Geometry: final body of the model. Coordinates: model frame, mm. Face numbers are marked on the shaded views. A direction names the side the tool comes from. Round coordinates to 2 decimals unless told otherwise and drop trailing zeros. Loops run counter-clockwise (first coordinate to the right, second up) from the corner with the lowest first, then second, coordinate; pieces in that order, holes last. Notation, with made-up numbers: M -4.5,71.5 L 33.5,71.5 A12 ccw 33.5,87.5 Z; hole C 5.25,53 d3. An arc over 180 degrees is marked long. Answer as a JSON object with one key per item and string values.
from build123d import *

# Parameters (mm, degrees)
F1_DEPTH = 6.35


with BuildPart() as f1:
    # F0 (on Front) → F1 (new body)
    with BuildSketch(Plane.XZ):
        with BuildLine():
            Line((52.175445, 0), (0, 0))
            ThreePointArc((0, 0), (-4.7752, -4.7752), (0, -9.5504))
            Line((0, -9.5504), (52.175445, -9.5504))
            ThreePointArc((52.175445, -9.5504), (54.631508, -10.044612), (56.705267, -11.45032))
            ThreePointArc((56.705267, -11.45032), (63.5, -14.3002), (70.294733, -11.45032))
            ThreePointArc((70.294733, -11.45032), (70.729047, -10.49401), (70.294733, -9.5377))
            Line((70.294733, -9.5377), (63.5, -9.5377))
            ThreePointArc((63.5, -9.5377), (58.7375, -4.7752), (63.5, -0.0127))
            Line((63.5, -0.0127), (70.294733, -0.0127))
            ThreePointArc((70.294733, -0.0127), (70.729047, 0.94361), (70.294733, 1.89992))
            ThreePointArc((70.294733, 1.89992), (63.5, 4.7498), (56.705267, 1.89992))
            ThreePointArc((56.705267, 1.89992), (54.631508, 0.494212), (52.175445, 0))
        make_face()
    extrude(amount=F1_DEPTH)


solid = f1.part
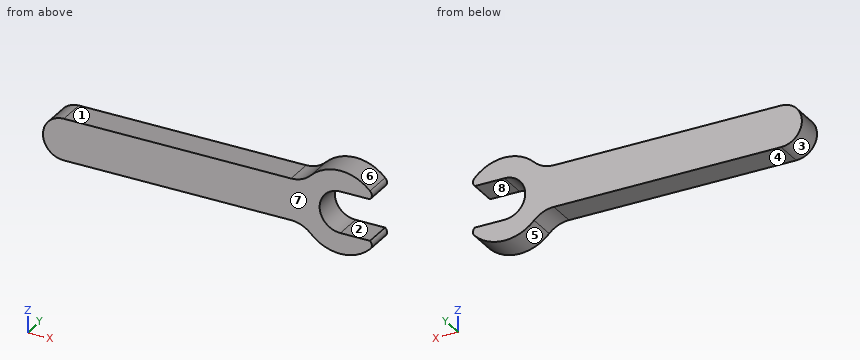
1) Ray query, line 1 (Z direction, x = 64, y = -1.75); line 2 (Z direction, x = 5, y = -0.75); line 3 (Z direction, x = 61, y = -3.5). Return the intervals inside material, ascending.
Results:
{"line 1": "-14.29 to -9.54, -0.01 to 4.74", "line 2": "-9.55 to 0", "line 3": "-13.97 to -8.83, -0.72 to 4.42"}
2) Pull-direction query (Z, two-part tool) for the marked faces 6, 7 and 8; classes: +Z half, -Z half, draft (parallel to the pull), parting line (faces both ways), or undercut.
Results:
{"face 6": "+Z half", "face 7": "draft", "face 8": "undercut"}
3) Reachability of the marked faces 1, 2, 3, 4 and 5 from +Z, -Z, +X, -X, +Y, -Y: full face, straight path, thin tool, end or side. Return the list, or none.
Results:
{"face 1": "+Z, -X, +Y, -Y", "face 2": "+X, +Y, -Y", "face 3": "-X, +Y, -Y", "face 4": "-Z, -X, +Y, -Y", "face 5": "-Z, +Y, -Y"}
4) Section query A-A (x = 62). Return the cut outline in (y, z).
Results:
{"outline": "M -6.35,-14.18 L 0,-14.18 L 0,-9.3 L -6.35,-9.3 Z; M -6.35,-0.26 L 0,-0.26 L 0,4.63 L -6.35,4.63 Z"}
5) Section query C-C (x = 10). Return the cut outline in (y, z).
Results:
{"outline": "M -6.35,-9.55 L 0,-9.55 L 0,0 L -6.35,0 Z"}
6) Pin query (flat end, axial travel): P1, Ø3, axis at x = 37.5, y = -3.5, coming from the +Z side; P2, Ø3, axis at x = 18.5, y = -0.5, coming from the -Z side; P3, Ø1.9, axis at x = 66.5, y = -4.5, coming from the +Z side; P4, Ø4, axis at x = 7.5, z = -5.5, coming from the +Y side. Return the tip coordinate at first contact, or that it passes through.
Results:
{"P1": "z = 0", "P2": "z = -9.55", "P3": "z = 4.53", "P4": "y = 0"}
